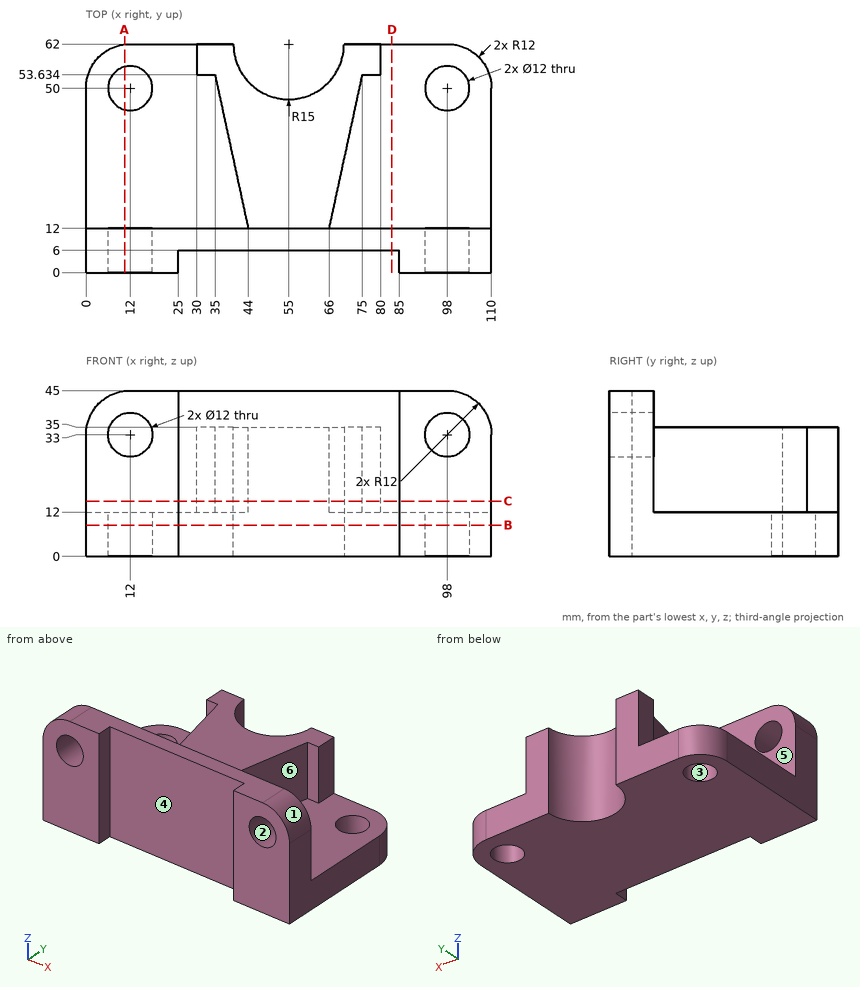
Answer from the drawing. Dimensions are ordinates in mm from the lowest x, y and z of the part. A direction names the side the tool comes from. Coordinates: 2 decimals unless noted, no trailing zeros. Loops run counter-clockwise (first coordinate to the right, second up) from the corner with the lowest first, then second, coordinate; pieces in that order, holes last. Notation, with made-up numbers: (80, 81.5) - (86, 81.5) arc R33 cw to (86, 119.5) - close; hole circle Ø9 at (-20.5, 6). An arc over 180 degrees is marked (long way). Use a Markdown table: item, result.
Item 1: Find section D-D, the plane x = 83. Determine the outline of the cut face in (y, z).
Evaluation:
| item | result |
|---|---|
| outline | (6, 0) - (62, 0) - (62, 12) - (12, 12) - (12, 45) - (6, 45) - close |
Item 2: Find section C-C, the plane z = 15. Determine the outline of the cut face in (x, y) (1 decimal), and give its area (3 significant figures).
Evaluation:
| item | result |
|---|---|
| outline | (0, 0) - (25, 0) - (25, 6) - (85, 6) - (85, 0) - (110, 0) - (110, 12) - (66, 12) - (75, 53.6) - (80, 53.6) - (80, 62) - (70, 62) arc R15 cw to (40, 62) - (30, 62) - (30, 53.6) - (35, 53.6) - (44, 12) - (0, 12) - close |
| area | 2,320 mm2 |
Item 3: Consider probe 1 along X at (y, z) = (7.5, 33); probe 2 along Y at (x, z) = (98, 3.5); probe 3 along X at (y, z) = (4, 33). Determine where each line is inside the solid, lowest interval first. Write a range as from..to.
Evaluation:
| item | result |
|---|---|
| probe 1 | x = 0..6, 18..92, 104..110 |
| probe 2 | y = 0..44, 56..62 |
| probe 3 | x = 0..6, 18..25, 85..92, 104..110 |
Item 4: The mould has two halves that part along Z. Classify the marked faces 1, 2 and 3: +Z half, -Z half, draft (parallel to the pull), parting line (faces both ways), or undercut.
Evaluation:
| item | result |
|---|---|
| face 1 | +Z half |
| face 2 | undercut |
| face 3 | draft |
Item 5: Find section A-A, the plane x = 10.5. Determine the outline of the cut face in (y, z), and give its area (3 significant figures).
Evaluation:
| item | result |
|---|---|
| outline | (0, 0) - (44.19, 0) - (44.19, 12) - (12, 12) - (12, 27.19) - (0, 27.19) - close; (0, 38.81) - (12, 38.81) - (12, 44.91) - (0, 44.91) - close; (55.81, 0) - (61.91, 0) - (61.91, 12) - (55.81, 12) - close |
| area | 859 mm2 |
Item 6: For the marked faces 4, 5 and 6, determine the directions among +Z, -Z, +X, -X, +Y, -Y from which every point of the face is accessible in a straight line to the end or side of a thin tool.
Evaluation:
| item | result |
|---|---|
| face 4 | +Z, -Z, -Y |
| face 5 | +Z |
| face 6 | +Z, +X |
Item 7: Given pin 1 Ø2.5 at (y, z) = (57, 29) entering from -X; pin 2 Ø13 at (x, y) = (15, 24.5) entering from +Z; pin 3 Ø2.5 at (y, z) = (58, 20.5) entering from +X; pin 4 Ø9.5 at (x, y) = (98, 50) entering from -Z, each flat-ended and moving along its own axis, determine where each tip first touches the part or whether it passes through.
Evaluation:
| item | result |
|---|---|
| pin 1 | stops at x = 30 |
| pin 2 | stops at z = 12 |
| pin 3 | stops at x = 80 |
| pin 4 | passes through |
Item 8: Find section B-B, the plane z = 8.5. Determine the outline of the cut face in (x, y), and give its area (3 significant figures).
Evaluation:
| item | result |
|---|---|
| outline | (0, 0) - (25, 0) - (25, 6) - (85, 6) - (85, 0) - (110, 0) - (110, 50) arc R12 ccw to (98, 62) - (70, 62) arc R15 cw to (40, 62) - (12, 62) arc R12 ccw to (0, 50) - close; hole circle Ø12 at (12, 50); hole circle Ø12 at (98, 50) |
| area | 5,820 mm2 |
